Autodesk Inventor part; units mm, degrees
ref_plane "YZ Plane" through (0, 0, 0) normal (1, 0, 0) x (0, 1, 0)
ref_plane "XZ Plane" through (0, 0, 0) normal (0, 1, 0) x (-1, 0, 0)
ref_plane "XY Plane" through (0, 0, 0) normal (0, 0, 1) x (1, 0, 0)
sketch "Sketch1" plane through (0, 0, 0) normal (0, 0, 1) x (1, 0, 0)
  circle A0 centre (0, 0) radius 6.35
  circle A1 centre (0, 0) radius 14.2875
  circle A2 centre (0, 0) radius 15.8623
  circle A3 centre (0, 0) radius 7.62
  circle A4 centre (0, 0) radius 13.0175
  dimension "d0" = 12.7
  dimension "d1" = 28.575
  dimension "d2" = 31.7246
  dimension "d7" = 15.24
  dimension "d8" = 26.035
extrude "Extrusion1" add sketch "Sketch1" along normal blind 7.112 contours A1 | A3 | A4
extrude "Extrusion2" add sketch "Sketch1" along normal blind 1.5748 contours A2
extrude "Extrusion3" cut sketch "Sketch1" along normal blind 0.635 contours A4
sketch "Sketch2" plane through (0, 0, 7.112) normal (0, 0, 1) x (1, 0, 0)
  circle A0 centre (0, 0) radius 7.62
  circle A1 centre (0, 0) radius 13.0175
extrude "Extrusion4" cut sketch "Sketch2" against normal blind 0.635
properties part number ".5 id 1.125 od flange bearing"
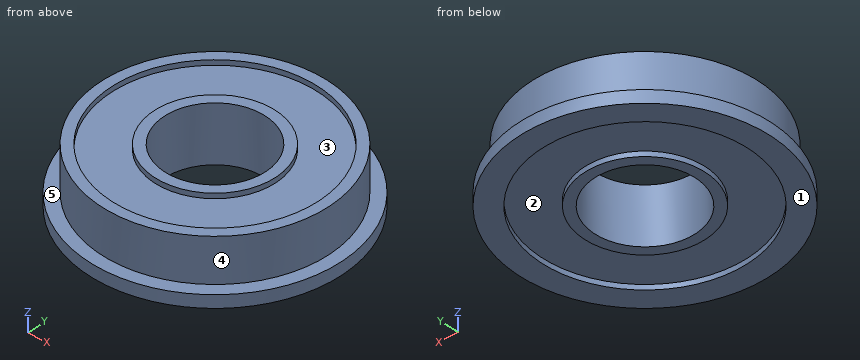
Build history of the part. All positions in model axes, mm. Face numbers are marked on the shaded views. A direction names the side the tool comes from. Coordinates: 2 decimals unless noted, no trailing zeros. Order: outer loops, then holes, each group sorted by start corner. A loop starts at its lowest first (then second) coordinate and runs counter-clockwise, first axis right, second up. Notation, with made-up numbers: M 23,87 L 27,87 A37 ccw 27,123 Z; hole C 11,-4.75 d1. An arc over 180 degrees is marked long. One line per question, with ' | ' between items. Start each with the question number.
Q1. Saw through at D-D (x = 9). List the corners of the cut face in (y, z) (3 decimals).
Q2. 3-axis set-ups, long thin cutter, end or side, ignore diameter. For the marked faces 1 and 2: which of +Z, -Z, +X, -X, +Y, -Y reach the whole face in a straight line?
Q3. Flat gauge pins, fed straight in: pin 1 Ø1 at (x, y) = (-3, 11) entering from -Z (3 decimals); pin 2 Ø3 at (x, z) = (6.5, 1.5) entering from +Y. Where does each tip first touch, or does it go through?
Q4. Two-plate mould, pull along Y, no slides. Class the marked faces 3, 4 and 5: +Y half, -Y half, draft (parallel to the pull), parting line (faces both ways), or undercut.
Q5. Probe L1, parallel to Y at x = 0, z = 0.4; L2, parallel to Y at x = 0, z = 2.5; L3, parallel to X at y = 4.5, z = 6.75. List the from-to ranges inside material, lowest first. Write a range as from..to.
Q6. Saw through at C-C (z = 1). List the corners of the cut face in (x, y), then the cut area to 3 significant figures.
Check values:
1) outline: M -13.062,0 L -9.405,0 L -9.405,0.635 L 9.405,0.635 L 9.405,0 L 13.062,0 L 13.062,1.575 L 11.097,1.575 L 11.097,7.112 L 9.405,7.112 L 9.405,6.477 L -9.405,6.477 L -9.405,7.112 L -11.097,7.112 L -11.097,1.575 L -13.062,1.575 Z
2) face 1: -Z, +X, -X, +Y, -Y | face 2: -Z
3) pin 1: stops at z = 0.635 | pin 2: stops at y = 15.05
4) face 3: undercut | face 4: parting line | face 5: draft
5) L1: y = -15.86..-13.02, -7.62..-6.35, 6.35..7.62, 13.02..15.86 | L2: y = -14.29..-6.35, 6.35..14.29 | L3: x = -13.56..-12.21, -6.15..-4.48, 4.48..6.15, 12.21..13.56
6) outline: C 0,0 d31.72; hole C 0,0 d12.7 | area: 664 mm2
